from build123d import *

# Parameters (mm, degrees)
F0_R         = 11.049
F1_DEPTH     = 6.35
F2_T2_ANGLE  = 120
F2_T4_ANGLE  = 240
F2_T6_ANGLE  = 120
F2_T8_ANGLE  = 240
F2_T10_ANGLE = 120
F2_T12_ANGLE = 240
F2_T22_ANGLE = 120
F2_T24_ANGLE = 240
F2_T26_ANGLE = 120
F2_T28_ANGLE = 240
F2_T30_ANGLE = 120
F2_T32_ANGLE = 240


# Not quite as in the source:
# - a fillet or chamfer that OpenCascade refuses, or shapes differently, is made with other operations: its cross-section is extruded or revolved along the edge and cut away or added


with BuildPart() as f1:
    # F0 (on Top) → F1 (new body)
    with BuildSketch(Plane.XY):
        with BuildLine():
            ThreePointArc((26.3964543073, 0), (13.1982271537, 7.62), (13.1982271537, 22.86))
            ThreePointArc((13.1982271537, 22.86), (0, 45.72), (-13.1982271537, 22.86))
            ThreePointArc((-13.1982271537, 22.86), (-13.1982271537, 7.62), (-26.3964543073, 0))
            ThreePointArc((-26.3964543073, 0), (-39.594681461, -22.86), (-13.1982271537, -22.86))
            ThreePointArc((-13.1982271537, -22.86), (0, -15.24), (13.1982271537, -22.86))
            ThreePointArc((13.1982271537, -22.86), (39.594681461, -22.86), (26.3964543073, 0))
        make_face()
        with Locations((-26.3964543073, -15.24)):
            Circle(F0_R, mode=Mode.SUBTRACT)
        with Locations((26.3964543073, -15.24)):
            Circle(F0_R, mode=Mode.SUBTRACT)
        with BuildLine():
            ThreePointArc((0, 11.049), (7.8128228253, 7.8128228253), (11.049, 0))
            ThreePointArc((11.049, 0), (-7.8128228253, -7.8128228253), (0, 11.049))
        make_face(mode=Mode.SUBTRACT)
        with Locations((0, 30.48)):
            Circle(F0_R, mode=Mode.SUBTRACT)
    extrude(amount=F1_DEPTH)

    # F2: chamfer of 2.54 on 20 edges, made by hand

    # F2_s1 → F2_t2 (revolve, cut)
    with BuildSketch(Plane.YZ.offset(26.3964543073)):
        Polygon((0, 3.81), (-2.54, 6.35), (0, 6.35), align=None)
    revolve(axis=Axis((26.3964543073, 15.24, 6.35), (0, 0, -1)), revolution_arc=F2_T2_ANGLE, mode=Mode.SUBTRACT)

    # F2_s3 → F2_t4 (revolve, cut)
    with BuildSketch(Plane(origin=(13.1982271537, 22.86, 0), x_dir=(0, 0, 1), z_dir=(-0.5, -0.8660254038, 0))):
        Polygon((6.35, 2.54), (3.81, 0), (6.35, 0), align=None)
    revolve(axis=Axis((0, 30.48, 6.35), (0, 0, 1)), revolution_arc=F2_T4_ANGLE, mode=Mode.SUBTRACT)

    # F2_s5 → F2_t6 (revolve, cut)
    with BuildSketch(Plane(origin=(-13.1982271537, 22.86, 0), x_dir=(0, 0, 1), z_dir=(-0.5, 0.8660254038, 0))):
        Polygon((6.35, 2.54), (3.81, 0), (6.35, 0), align=None)
    revolve(axis=Axis((-26.3964543073, 15.24, 6.35), (0, 0, -1)), revolution_arc=F2_T6_ANGLE, mode=Mode.SUBTRACT)

    # F2_s7 → F2_t8 (revolve, cut)
    with BuildSketch(Plane.YZ.offset(-26.3964543073)):
        Polygon((-2.54, 6.35), (0, 3.81), (0, 6.35), align=None)
    revolve(axis=Axis((-26.3964543073, -15.24, 6.35), (0, 0, 1)), revolution_arc=F2_T8_ANGLE, mode=Mode.SUBTRACT)

    # F2_s9 → F2_t10 (revolve, cut)
    with BuildSketch(Plane(origin=(-13.1982271537, -22.86, 0), x_dir=(0, 0, 1), z_dir=(-0.5, -0.8660254038, 0))):
        Polygon((6.35, 2.54), (3.81, 0), (6.35, 0), align=None)
    revolve(axis=Axis((0, -30.48, 6.35), (0, 0, -1)), revolution_arc=F2_T10_ANGLE, mode=Mode.SUBTRACT)

    # F2_s11 → F2_t12 (revolve, cut)
    with BuildSketch(Plane(origin=(13.1982271537, -22.86, 0), x_dir=(0, 0, 1), z_dir=(-0.5, 0.8660254038, 0))):
        Polygon((6.35, 2.54), (3.81, 0), (6.35, 0), align=None)
    revolve(axis=Axis((26.3964543073, -15.24, 6.35), (0, 0, 1)), revolution_arc=F2_T12_ANGLE, mode=Mode.SUBTRACT)

    # F2_s13 → F2_t14 (revolve, cut)
    with BuildSketch(Plane.XZ.offset(15.24)):
        Polygon((-12.8074543073, 6.35), (-15.3474543073, 3.81), (-15.3474543073, 6.35), align=None)
    revolve(axis=Axis((-26.3964543073, -15.24, 6.35), (0, 0, 1)), mode=Mode.SUBTRACT)

    # F2_s15 → F2_t16 (revolve, cut)
    with BuildSketch(Plane.XZ.offset(15.24)):
        Polygon((39.9854543073, 6.35), (37.4454543073, 3.81), (37.4454543073, 6.35), align=None)
    revolve(axis=Axis((26.3964543073, -15.24, 6.35), (0, 0, 1)), mode=Mode.SUBTRACT)

    # F2_s17 → F2_t18 (revolve, cut)
    with BuildSketch(Plane.YZ):
        Polygon((13.589, 6.35), (11.049, 3.81), (11.049, 6.35), align=None)
    revolve(axis=Axis((0, 0, 6.35), (0, 0, 1)), mode=Mode.SUBTRACT)

    # F2_s19 → F2_t20 (revolve, cut)
    with BuildSketch(Plane.XZ.offset(-30.48)):
        Polygon((13.589, 6.35), (11.049, 3.81), (11.049, 6.35), align=None)
    revolve(axis=Axis((0, 30.48, 6.35), (0, 0, 1)), mode=Mode.SUBTRACT)

    # F2_s21 → F2_t22 (revolve, cut)
    with BuildSketch(Plane.YZ.offset(26.3964543073)):
        Polygon((0, 2.54), (-2.54, 0), (0, 0), align=None)
    revolve(axis=Axis((26.3964543073, 15.24, 0), (0, 0, -1)), revolution_arc=F2_T22_ANGLE, mode=Mode.SUBTRACT)

    # F2_s23 → F2_t24 (revolve, cut)
    with BuildSketch(Plane(origin=(13.1982271537, 22.86, 0), x_dir=(0, 0, 1), z_dir=(-0.5, -0.8660254038, 0))):
        Polygon((0, 2.54), (2.54, 0), (0, 0), align=None)
    revolve(axis=Axis((0, 30.48, 0), (0, 0, 1)), revolution_arc=F2_T24_ANGLE, mode=Mode.SUBTRACT)

    # F2_s25 → F2_t26 (revolve, cut)
    with BuildSketch(Plane(origin=(-13.1982271537, 22.86, 0), x_dir=(0, 0, 1), z_dir=(-0.5, 0.8660254038, 0))):
        Polygon((2.54, 0), (0, 2.54), (0, 0), align=None)
    revolve(axis=Axis((-26.3964543073, 15.24, 0), (0, 0, -1)), revolution_arc=F2_T26_ANGLE, mode=Mode.SUBTRACT)

    # F2_s27 → F2_t28 (revolve, cut)
    with BuildSketch(Plane.YZ.offset(-26.3964543073)):
        Polygon((0, 2.54), (-2.54, 0), (0, 0), align=None)
    revolve(axis=Axis((-26.3964543073, -15.24, 0), (0, 0, 1)), revolution_arc=F2_T28_ANGLE, mode=Mode.SUBTRACT)

    # F2_s29 → F2_t30 (revolve, cut)
    with BuildSketch(Plane(origin=(-13.1982271537, -22.86, 0), x_dir=(0, 0, 1), z_dir=(-0.5, -0.8660254038, 0))):
        Polygon((2.54, 0), (0, 2.54), (0, 0), align=None)
    revolve(axis=Axis((0, -30.48, 0), (0, 0, -1)), revolution_arc=F2_T30_ANGLE, mode=Mode.SUBTRACT)

    # F2_s31 → F2_t32 (revolve, cut)
    with BuildSketch(Plane(origin=(13.1982271537, -22.86, 0), x_dir=(0, 0, 1), z_dir=(-0.5, 0.8660254038, 0))):
        Polygon((0, 2.54), (2.54, 0), (0, 0), align=None)
    revolve(axis=Axis((26.3964543073, -15.24, 0), (0, 0, 1)), revolution_arc=F2_T32_ANGLE, mode=Mode.SUBTRACT)

    # F2_s33 → F2_t34 (revolve, cut)
    with BuildSketch(Plane.XZ.offset(15.24)):
        Polygon((-15.3474543073, 2.54), (-12.8074543073, 0), (-15.3474543073, 0), align=None)
    revolve(axis=Axis((-26.3964543073, -15.24, 0), (0, 0, 1)), mode=Mode.SUBTRACT)

    # F2_s35 → F2_t36 (revolve, cut)
    with BuildSketch(Plane.XZ.offset(15.24)):
        Polygon((37.4454543073, 2.54), (39.9854543073, 0), (37.4454543073, 0), align=None)
    revolve(axis=Axis((26.3964543073, -15.24, 0), (0, 0, 1)), mode=Mode.SUBTRACT)

    # F2_s37 → F2_t38 (revolve, cut)
    with BuildSketch(Plane.YZ):
        Polygon((11.049, 2.54), (13.589, 0), (11.049, 0), align=None)
    revolve(axis=Axis((0, 0, 0), (0, 0, -1)), mode=Mode.SUBTRACT)

    # F2_s39 → F2_t40 (revolve, cut)
    with BuildSketch(Plane.XZ.offset(-30.48)):
        Polygon((11.049, 2.54), (13.589, 0), (11.049, 0), align=None)
    revolve(axis=Axis((0, 30.48, 0), (0, 0, 1)), mode=Mode.SUBTRACT)


solid = f1.part
Read the model definition and answer for the solid it produces. Units are mm, in the model's axes. Give positions to 0.01 mm unless a question says otherwise; leave off trailing zeros. Loops run counter-clockwise (first coordinate to the right, second up) from the corner with the lowest first, then second, coordinate; pieces in that order, holes last. Notation, with made-up numbers: (85.25, 87) -> (130.25, 87) arc R11 cw to (130.25, 91) -> close; hole circle Ø6 at (60, 41.5). An arc over 180 degrees is marked (long way). Answer as CSV lines item,"result".
Item 1: Determine the mould class of faces 1 (the face through (13, -8, 6.35)), 2 (the face through (-15.86, -11.92, 3.17)) for opening direction Y: +Y half, -Y half, draft (parallel to the pull), parting line (faces both ways), or undercut.
Returned:
face 1,"draft"
face 2,"undercut"
Item 2: Find section B-B on x = -7.5. State how many separate pieces and enclosed holes the cut face has, plus the area to 3 significant figures.
Returned:
separate pieces,"3"
enclosed holes,"0"
area,"133 mm²"
Item 3: Find section A-A on y = 30.48. Give the vertices of the cut face in (x, z).
Returned:
outline,"(-15.24, 2.54) -> (-13.14, 0.44) -> (-11.05, 2.54) -> (-11.05, 3.81) -> (-13.14, 5.91) -> (-15.24, 3.81) -> close; (11.05, 2.54) -> (13.14, 0.44) -> (15.24, 2.54) -> (15.24, 3.81) -> (13.14, 5.91) -> (11.05, 3.81) -> close"
Item 4: Each of these flat-tipped pins is pushed along its axis until it touches: pin 1 (10 mm diameter, centred on x = 6, y = 7.5, fed in from +Z); pin 2 (20 mm diameter, centred on x = 0, y = 0, fed in from +Z); pin 3 (1.5 mm diameter, centred on y = 35.5, z = 3.5, fed in from -X); pin 4 (1 mm diameter, centred on x = 7, z = 4, fed in from +Y). Where does it stop, or does it pass through?
Returned:
pin 1,"stops at z = 6.35"
pin 2,"passes through"
pin 3,"stops at x = -14.63"
pin 4,"stops at y = 44.25"
Item 5: Consider line 1 (Y direction, x = 0, z = 3.2); line 2 (Y direction, x = 0.5, z = 1.5); line 3 (X direction, y = -5, z = 1). Determine where each line is inside the solid, lowest interval first. Write a range as [from, to].
Returned:
line 1,"y = [-15.24, -11.05], [11.05, 19.43], [41.53, 45.72]"
line 2,"y = [-14.21, -12.08], [12.08, 18.4], [42.56, 44.67]"
line 3,"x = [-35.5, -33.72], [-19.07, -11.55], [11.55, 19.07], [33.72, 35.5]"
